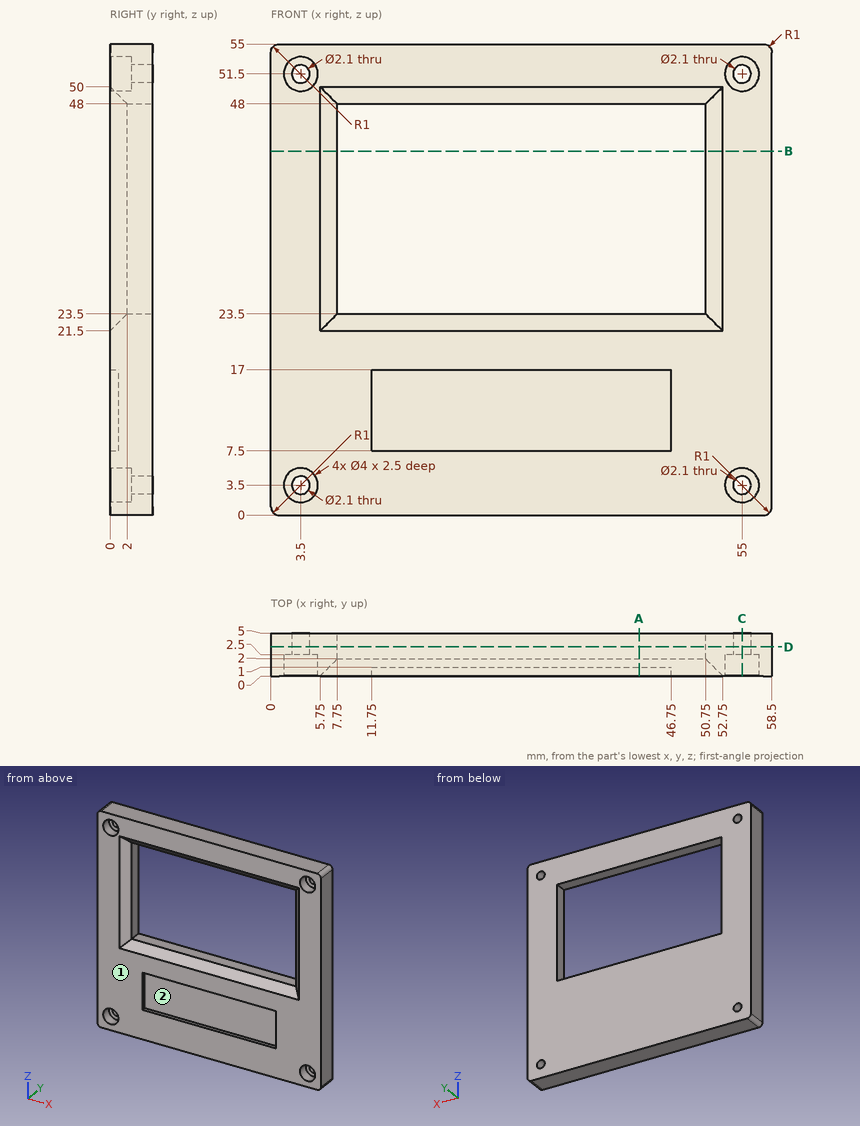
Geometry: see drawing. Coordinates: mm, zero at the bounding-box minimum. Give positions to 0.01 mm unless a question says otherwise; leave off trailing zeros. Loops run counter-clockwise (first coordinate to the right, second up) from the corner with the lowest first, then second, coordinate; pieces in that order, holes last. Notation, with made-up numbers: (-38, 64) - (1, 64) arc R20 ccw to (1, 89) - close; hole circle Ø1 at (55.25, -27.5). An arc over 180 degrees is marked (long way). One line per question, with ' | ' between items. Start each with the question number.
(1) Contact query for flat-ended pins moving along their axis: pin 1 (3.5 mm diameter, centred on x = 55, z = 51.5, fed in from -Y); pin 2 (7.5 mm diameter, centred on x = 34, z = 13, fed in from -Y); pin 3 (8 mm diameter, centred on x = 23, z = 26, fed in from -Y). Output: stop coordinate, or through.
(2) Section query A-A on x = 43. Return loops of the section in (y, z), then the cut area to 3 significant figures.
(3) Pull-direction query (Z, two-part tool) for the marked faces 1 and 2; classes: released by +Z, released by -Z, zero draft, split by the parting line, or undercut.
(4) Section query B-B on z = 42.5. Return loops of the section in (x, y), then the cut area to 3 significant figures.
(5) Section query C-C on x = 55. Return loops of the section in (y, z), then the cut area to 4 significant figures.
(6) Ray query, line 1 (Z direction, x = 55, y = 1.55); line 2 (X direction, y = 4.4, z = 38.5); line 3 (Z direction, x = 9, y = 4.75). Return the intervals inside material, ascending. Write a range as from..to.
(7) Section query D-D on y = 3.4. Return loops of the section in (x, z).
The answers:
1) pin 1: y = 2.5 | pin 2: y = 1 | pin 3: y = 0.5
2) outline: (0, 0) - (5, 0) - (5, 23.5) - (2, 23.5) - (0, 21.5) - (0, 17) - (1, 17) - (1, 7.5) - (0, 7.5) - close; (0, 50) - (2, 48) - (5, 48) - (5, 55) - (0, 55) - close | area: 139 mm2
3) face 1: zero draft | face 2: undercut
4) outline: (0, 0) - (5.75, 0) - (7.75, 2) - (7.75, 5) - (0, 5) - close; (50.75, 2) - (52.75, 0) - (58.5, 0) - (58.5, 5) - (50.75, 5) - close | area: 73.5 mm2
5) outline: (0, 0) - (5, 0) - (5, 2.45) - (2.5, 2.45) - (2.5, 1.5) - (0, 1.5) - close; (0, 5.5) - (2.5, 5.5) - (2.5, 4.55) - (5, 4.55) - (5, 50.45) - (2.5, 50.45) - (2.5, 49.5) - (0, 49.5) - close; (0, 53.5) - (2.5, 53.5) - (2.5, 52.55) - (5, 52.55) - (5, 55) - (0, 55) - close | area: 244.5 mm2
6) line 1: 0..1.5, 5.5..49.5, 53.5..55 | line 2: 0..7.75, 50.75..58.5 | line 3: 0..23.5, 48..55
7) outline: (0, 1) arc R1 ccw to (1, 0) - (57.5, 0) arc R1 ccw to (58.5, 1) - (58.5, 54) arc R1 ccw to (57.5, 55) - (1, 55) arc R1 ccw to (0, 54) - close; hole circle Ø2.1 at (3.5, 3.5); hole circle Ø2.1 at (3.5, 51.5); hole (7.75, 23.5) - (50.75, 23.5) - (50.75, 48) - (7.75, 48) - close; hole circle Ø2.1 at (55, 3.5); hole circle Ø2.1 at (55, 51.5)
